from build123d import *

# Parameters (mm, degrees)
SKETCH_1_W          = 103
SKETCH_1_H          = 61.2
EXTRUDE_1_DEPTH     = 3
SKETCH_2_R          = 1.5
SKETCH_2_R_2        = 1.525
CUT_EXTRUDE_1_DEPTH = 10
SKETCH_3_W          = 83
SKETCH_3_H          = 28.4
SKETCH_3_R          = 1.55
EXTRUDE_2_DEPTH     = 3
CUT_EXTRUDE_5_DEPTH = 10
FILLET_1_R          = 2
CUT_EXTRUDE_2_DEPTH = 10
FILLET_3_R          = 2
CUT_EXTRUDE_3_DEPTH = 10
EXTRUDE_3_DEPTH     = 3
FILLET_2_R          = 2
CUT_EXTRUDE_4_DEPTH = 10
FILLET_4_R          = 3
FILLET_6_R          = 6
SKETCH_11_W         = 4
SKETCH_11_H         = 82.358538581
EXTRUDE_4_DEPTH     = 3
FILLET_7_R          = 2


with BuildPart() as part:
    # 草图1 → 凸台-拉伸1 (new body)
    with BuildSketch(Plane.XY):
        Rectangle(SKETCH_1_W, SKETCH_1_H)
    extrude(amount=EXTRUDE_1_DEPTH)

    # 草图2 → 切除-拉伸1 (cut)
    with BuildSketch(Plane(origin=(0, 0, 0), x_dir=(-1, 0, 0), z_dir=(0, 0, -1))):
        with Locations((-42.5, 27.6)):
            Circle(SKETCH_2_R)
        with Locations((-42.5, -27.6)):
            Circle(SKETCH_2_R)
        with Locations((42.499997562, -27.6)):
            Circle(SKETCH_2_R)
        with Locations((42.499997562, 27.6)):
            Circle(SKETCH_2_R)
        with Locations((32, 27.6)):
            Circle(SKETCH_2_R_2)
        with Locations((32, 19.6)):
            Circle(SKETCH_2_R_2)
        Polygon((-39.5, 22.074667925), (-39.5, -22.074667925), (-5.508211597, 0), align=None)
        Polygon((-1.219e-06, -2.38473115), (-35.748149691, -25.6), (35.748147253, -25.6), align=None)
        Polygon((39.499997562, 22.074667925), (5.50820916, 0), (39.499997562, -22.074667925), align=None)
        with BuildLine():
            Line((-43.5, 19.6), (-43.5, -19.059996805))
            ThreePointArc((-43.5, -19.059996805), (-46, -21.559996805), (-48.5, -19.059996805))
            Line((-48.5, -19.059996805), (-48.5, 19.6))
            ThreePointArc((-48.5, 19.6), (-46, 22.1), (-43.5, 19.6))
        make_face()
        with BuildLine():
            Line((43.5, 19.6), (43.5, -19.059996805))
            ThreePointArc((43.5, -19.059996805), (46, -21.559996805), (48.5, -19.059996805))
            Line((48.5, -19.059996805), (48.5, 19.6))
            ThreePointArc((48.5, 19.6), (46, 22.1), (43.5, 19.6))
        make_face()
    extrude(amount=-CUT_EXTRUDE_1_DEPTH, mode=Mode.SUBTRACT)

    # 草图3 → 凸台-拉伸2 (add)
    with BuildSketch(Plane.XY.offset(3)):
        with Locations((0.4, -44.8)):
            Rectangle(SKETCH_3_W, SKETCH_3_H)
        with Locations((-37.1, -33)):
            Circle(SKETCH_3_R, mode=Mode.SUBTRACT)
        with Locations((-37.1, -55)):
            Circle(SKETCH_3_R, mode=Mode.SUBTRACT)
        with Locations((37.9, -55)):
            Circle(SKETCH_3_R, mode=Mode.SUBTRACT)
        with Locations((37.9, -33)):
            Circle(SKETCH_3_R, mode=Mode.SUBTRACT)
    extrude(amount=-EXTRUDE_2_DEPTH)

    # 草图10 → 切除-拉伸5 (cut)
    with BuildSketch(Plane(origin=(0, 0, 0), x_dir=(-1, 0, 0), z_dir=(0, 0, -1))):
        Polygon((-39.124074846, 26.6), (27, 26.6), (27, 18.726482933), (0, 1.192364783), align=None)
    extrude(amount=-CUT_EXTRUDE_5_DEPTH, mode=Mode.SUBTRACT)

    # 圆角1
    fillet_1_edges = [part.edges().sort_by_distance(p)[0] for p in [
        (0, 1.192364783, 1.5),
        (39.124074846, 26.6, 1.5),
        (-27, 26.6, 1.5),
        (-27, 18.726482933, 1.5),
        (-39.499997562, 22.074667925, 1.5),
        (-39.499997562, -22.074667925, 1.5),
        (-5.50820916, 0, 1.5),
        (1.219e-06, -2.38473115, 1.5),
        (-35.748147253, -25.6, 1.5),
        (35.748149691, -25.6, 1.5),
        (39.5, 22.074667925, 1.5),
        (5.508211597, 0, 1.5),
        (39.5, -22.074667925, 1.5),
        (-51.5, 30.6, 1.5),
        (51.5, 30.6, 1.5),
        (51.5, -30.6, 1.5),
        (-51.5, -30.6, 1.5),
    ]]
    fillet(fillet_1_edges, radius=FILLET_1_R)

    # 草图4 → 切除-拉伸2 (cut)
    with BuildSketch(Plane.XY.offset(3)):
        with BuildLine():
            ThreePointArc((-32.517424305, -35), (-33.564466094, -36.535533906), (-35.1, -37.582575695))
            Line((-35.1, -37.582575695), (-35.1, -50.417424305))
            ThreePointArc((-35.1, -50.417424305), (-33.564466094, -51.464466094), (-32.517424305, -53))
            Line((-32.517424305, -53), (33.317424305, -53))
            ThreePointArc((33.317424305, -53), (34.364466094, -51.464466094), (35.9, -50.417424305))
            Line((35.9, -50.417424305), (35.9, -37.582575695))
            ThreePointArc((35.9, -37.582575695), (34.364466094, -36.535533906), (33.317424305, -35))
            Line((33.317424305, -35), (-32.517424305, -35))
        make_face()
    extrude(amount=-CUT_EXTRUDE_2_DEPTH, mode=Mode.SUBTRACT)

    # 圆角3
    fillet_3_edges = [part.edges().sort_by_distance(p)[0] for p in [
        (35.9, -50.417424305, 1.5),
        (33.317424305, -53, 1.5),
        (-32.517424305, -53, 1.5),
        (-35.1, -50.417424305, 1.5),
        (-35.1, -37.582575695, 1.5),
        (-32.517424305, -35, 1.5),
        (33.317424305, -35, 1.5),
        (35.9, -37.582575695, 1.5),
    ]]
    fillet(fillet_3_edges, radius=FILLET_3_R)

    # 草图6 → 切除-拉伸3 (cut)
    with BuildSketch(Plane.XY.offset(3)):
        with BuildLine():
            Line((-40.999997562, 28.6), (-40.999997562, 24.6))
            ThreePointArc((-40.999997562, 24.6), (-42.499997562, 23.1), (-43.999997562, 24.6))
            Line((-43.999997562, 24.6), (-43.999997562, 28.6))
            ThreePointArc((-43.999997562, 28.6), (-42.499997562, 30.1), (-40.999997562, 28.6))
        make_face()
        with BuildLine():
            Line((-40.999997562, -28.6), (-40.999997562, -24.6))
            ThreePointArc((-40.999997562, -24.6), (-42.499997562, -23.1), (-43.999997562, -24.6))
            Line((-43.999997562, -24.6), (-43.999997562, -28.6))
            ThreePointArc((-43.999997562, -28.6), (-42.499997562, -30.1), (-40.999997562, -28.6))
        make_face()
        with BuildLine():
            Line((40.999997562, -28.6), (40.999997562, -24.6))
            ThreePointArc((40.999997562, -24.6), (42.499997562, -23.1), (43.999997562, -24.6))
            Line((43.999997562, -24.6), (43.999997562, -28.6))
            ThreePointArc((43.999997562, -28.6), (42.499997562, -30.1), (40.999997562, -28.6))
        make_face()
        with BuildLine():
            Line((40.999997562, 28.6), (40.999997562, 24.6))
            ThreePointArc((40.999997562, 24.6), (42.499997562, 23.1), (43.999997562, 24.6))
            Line((43.999997562, 24.6), (43.999997562, 28.6))
            ThreePointArc((43.999997562, 28.6), (42.499997562, 30.1), (40.999997562, 28.6))
        make_face()
    extrude(amount=-CUT_EXTRUDE_3_DEPTH, mode=Mode.SUBTRACT)

    # 草图7 → 凸台-拉伸3 (add)
    with BuildSketch(Plane.XY.offset(3)):
        with BuildLine():
            Line((39.035895947, 30.6), (45.964099177, 30.6))
            ThreePointArc((45.964099177, 30.6), (42.499997562, 32.6), (39.035895947, 30.6))
        make_face()
        with BuildLine():
            Line((-34.645751311, 30.6), (-29.354248689, 30.6))
            ThreePointArc((-29.354248689, 30.6), (-32, 31.6), (-34.645751311, 30.6))
        make_face()
        with BuildLine():
            ThreePointArc((41.9, -33.563869753), (44.982206885, -32.940349856), (47.082573257, -30.6))
            Line((47.082573257, -30.6), (41.9, -30.6))
            Line((41.9, -30.6), (41.9, -33.563869753))
        make_face()
        with BuildLine():
            Line((-45.964099177, 30.6), (-39.035895947, 30.6))
            ThreePointArc((-39.035895947, 30.6), (-42.499997562, 32.6), (-45.964099177, 30.6))
        make_face()
        with BuildLine():
            Line((-30.193716195, 16.031059146), (-35.995070346, 19.798526892))
            ThreePointArc((-35.995070346, 19.798526892), (-34.178566027, 16.245324149), (-30.193716195, 16.031059146))
        make_face()
        with BuildLine():
            ThreePointArc((-47.082573257, -30.6), (-44.619479076, -33.128553645), (-41.1, -33.400000711))
            Line((-41.1, -33.400000711), (-41.1, -30.6))
            Line((-41.1, -30.6), (-47.082573257, -30.6))
        make_face()
    extrude(amount=-EXTRUDE_3_DEPTH)

    # 圆角2
    fillet_2_edges = [part.edges().sort_by_distance(p)[0] for p in [
        (-41.1, -59, 1.5),
        (41.9, -59, 1.5),
        (-39.035895947, 30.6, 1.5),
        (-45.964099177, 30.6, 1.5),
        (45.964099177, 30.6, 1.5),
        (39.035895947, 30.6, 1.5),
    ]]
    fillet(fillet_2_edges, radius=FILLET_2_R)

    # 草图8 → 切除-拉伸4 (cut)
    with BuildSketch(Plane.XY.offset(3)):
        with BuildLine():
            Line((0, -31), (0, -2.384731941))
            Line((0, -2.384731941), (-38.011080882, -27.069575763))
            ThreePointArc((-38.011080882, -27.069575763), (-34.018985575, -27.851471073), (-31.443145751, -31))
            Line((-31.443145751, -31), (0, -31))
        make_face()
        with BuildLine():
            Line((37.903948732, -27.000001299), (0, -2.384731941))
            Line((0, -2.384731941), (0, -31))
            Line((0, -31), (32.243145751, -31))
            ThreePointArc((32.243145751, -31), (34.437510635, -28.099880879), (37.903948732, -27.000001299))
        make_face()
    extrude(amount=-CUT_EXTRUDE_4_DEPTH, mode=Mode.SUBTRACT)

    # 圆角4
    # the kernel refuses this fillet: 3 mm, written as the material it adds along each edge
    with BuildSketch(Plane(origin=(32.243145751, -31, 3), x_dir=(0.4479167728471886, 0.8940752566770652, 0), z_dir=(0, 0, -1))) as fillet_4_piece_1:
        with BuildLine():
            CenterArc((1.864123466, -2.97674348), FILLET_4_R, 97.138883981, 56.251011404)
            Line((-0.818102304, -1.632993162), (-0.871746819, -1.606118155))
            Line((-0.871746819, -1.606118155), (-0.053644515, 0.026875006))
            Line((-0.053644515, 0.026875006), (0.007456494, 0.05953487))
            ThreePointArc((0.007456494, 0.05953487), (0.745649387, 0.013486961), (1.483842279, 0.05953487))
            Line((1.483842279, 0.05953487), (1.491298773, 0))
        make_face()
    extrude(amount=3)
    with BuildSketch(Plane(origin=(-31.443145751, -31, 3), x_dir=(1, 0, 0), z_dir=(0, 0, -1))) as fillet_4_piece_2:
        with BuildLine():
            CenterArc((1.826460524, -3), FILLET_4_R, 90, 56.251011404)
            Line((-0.667977734, -1.333333333), (-0.717866499, -1.3))
            ThreePointArc((-0.717866499, -1.3), (-0.346047225, -0.660625631), (-0.056568542, 0.02))
            Line((-0.056568542, 0.02), (0, 0.06))
            Line((0, 0.06), (1.826460524, 0.06))
            Line((1.826460524, 0.06), (1.826460524, 0))
        make_face()
    extrude(amount=3)
    with BuildSketch(Plane(origin=(37.903948732, -27.000001299, 3), x_dir=(-0.8386689787810934, 0.5446414821056857, 0), z_dir=(0, 0, -1))) as fillet_4_piece_3:
        with BuildLine():
            CenterArc((5.502571293, -3), FILLET_4_R, 90, 103.062756756)
            Line((2.580202026, -3.678054475), (2.521754641, -3.691615565))
            ThreePointArc((2.521754641, -3.691615565), (1.598242731, -1.622861901), (-0.032645365, -0.050341634))
            Line((-0.032645365, -0.050341634), (0, 0.06))
            Line((0, 0.06), (5.502571293, 0.06))
            Line((5.502571293, 0.06), (5.502571293, 0))
        make_face()
    extrude(amount=3)
    with BuildSketch(Plane(origin=(-38.011080882, -27.069575763, 3), x_dir=(0.9604450270381002, -0.278469657301802, 0), z_dir=(0, 0, -1))) as fillet_4_piece_4:
        with BuildLine():
            CenterArc((6.316215768, -2.721069043), FILLET_4_R, 114.902857597, 105.92808325)
            Line((4.046289512, -4.682556945), (4.000890987, -4.721786703))
            Line((4.000890987, -4.721786703), (-0.045398525, -0.039229758))
            Line((-0.045398525, -0.039229758), (0.025264863, 0.054421381))
            ThreePointArc((0.025264863, 0.054421381), (2.526486307, -0.497861915), (5.027707751, 0.054421381))
            Line((5.027707751, 0.054421381), (5.052972614, 0))
        make_face()
    extrude(amount=3)
    with BuildSketch(Plane(origin=(0, -2.384731941, 3), x_dir=(-0.8386689627806916, -0.5446415067439856, 0), z_dir=(0, 0, -1))) as fillet_4_piece_5:
        with BuildLine():
            CenterArc((FILLET_4_R * 0.649411762447, -FILLET_4_R), FILLET_4_R, 90, 66.000336041)
            Line((-FILLET_4_R * 0.2641360807, -FILLET_4_R * 0.593268714899), (-FILLET_4_R * 0.282407037563, -FILLET_4_R * 0.585134089197))
            Line((-FILLET_4_R * 0.282407037563, -FILLET_4_R * 0.585134089197), (-FILLET_4_R * 0.0129882352489, FILLET_4_R * 0.02))
            Line((-FILLET_4_R * 0.0129882352489, FILLET_4_R * 0.02), (FILLET_4_R * 0.649411762447, FILLET_4_R * 0.02))
            Line((FILLET_4_R * 0.649411762447, FILLET_4_R * 0.02), (FILLET_4_R * 0.649411762447, 0))
        make_face()
    extrude(amount=3)

    # 圆角6
    fillet_6_edges = [part.edges().sort_by_distance(p)[0] for p in [
        (-47.082573257, -30.6, 1.5),
        (47.082573257, -30.6, 1.5),
        (41.9, -33.563869753, 1.5),
        (-41.1, -33.400000711, 1.5),
    ]]
    fillet(fillet_6_edges, radius=FILLET_6_R)

    # 草图11 → 凸台-拉伸4 (add)
    with BuildSketch(Plane.XY.offset(3)):
        with Locations((0, -14.579269291)):
            Rectangle(SKETCH_11_W, SKETCH_11_H)
    extrude(amount=-EXTRUDE_4_DEPTH)

    # 圆角7
    fillet_7_edges = [part.edges().sort_by_distance(p)[0] for p in [
        (-2, -31, 1.5),
        (2, -31, 1.5),
        (2, 26.6, 1.5),
        (2, -53, 1.5),
        (2, -3.683553925, 1.5),
        (2, 2.49118835, 1.5),
        (-2, -53, 1.5),
        (-2, -3.683555508, 1.5),
        (-2, 2.49118835, 1.5),
        (-2, 26.6, 1.5),
        (2, -35, 1.5),
        (-2, -35, 1.5),
    ]]
    fillet(fillet_7_edges, radius=FILLET_7_R)


solid = part.part
Geometry: final body of the model. Coordinates: model frame, mm. A direction names the side the tool comes from. Coordinates: 2 decimals unless noted, no trailing zeros. Order: outer loops, then holes, each group sorted by start corner. A loop starts at its lowest first (then second) coordinate and runs counter-clockwise, first axis right, second up. Notation, with made-up numbers: (49.5, -2) - (101.5, -2) arc R18 cw to (101.5, 32) - close; hole circle Ø4 at (29.5, 74.5). An arc over 180 degrees is marked (long way). Use one line per item in the form item = value.
1) Set-up query: faces 5 (the face through (-48, 30.6, 1)), 6 (the face through (-42.5, 23.1, 1.5)), 7 (the face through (0, -16, 3)). Return all of +Z, -Z, +X, -X, +Y, -Y with unobstructed straight access to the full face (end or side cutting, diameter ignored); none if empty.
Solutions:
face_5 = +Z, -Z, -X, +Y
face_6 = +Z, -Z
face_7 = +Z, +X, -X, +Y, -Y
2) Section B-B (z = 2.3). State how many separate pieces and enclosed holes the cut face has, then the cut area to 3 significant figures.
Solutions:
separate_pieces = 1
enclosed_holes = 20
area = 3,610 mm^2
3) Pin query (flat end, axial travel): pin 1 (1.5 mm diameter, centred on x = -36, z = 1, fed in from +Y). Return the tip coordinate at first contact, or that it passes through.
Solutions:
pin_1 = 30.6
4) Section A-A (x = 13.5). Return loops of the section in (y, z).
Solutions:
outline = (-59, 0) - (-53, 0) - (-53, 3) - (-59, 3) - close; (-35, 0) - (-31, 0) - (-31, 3) - (-35, 3) - close; (-11.15, 0) - (-5.19, 0) - (-5.19, 3) - (-11.15, 3) - close; (5.19, 0) - (9.96, 0) - (9.96, 3) - (5.19, 3) - close; (26.6, 0) - (30.6, 0) - (30.6, 3) - (26.6, 3) - close
5) Mould query, pull axis X, two halves, no side actions, for faces 1 (the face through (51.5, 0, 1)), 2 (the face through (42.5, -23.1, 1.5)), 3 (the face through (0, -59, 2)), 4 (the face through (-22.053, -10.744, 1.479)). Classes: +X half, -X half, draft (parallel to the pull), parting line (faces both ways), or undercut.
Solutions:
face_1 = +X half
face_2 = undercut
face_3 = draft
face_4 = undercut
6) Ray query, L1, parallel to Y at x = 21, z = 1.2; L2, parallel to Y at x = -3.5, z = 1; L3, parallel to Y at x = -21.5, z = 2.35. Return the intervals inside material, ascending.
Solutions:
L1 = -59 to -53, -35 to -31, -16.02 to -10.06, 10.06 to 14.83, 26.6 to 30.6
L2 = -59 to -52.94, -35.06 to -30.94, -5.43 to 4.24, 26.54 to 30.6
L3 = -59 to -53, -35 to -31, -16.35 to -10.39, 10.39 to 15.15, 26.6 to 30.6
